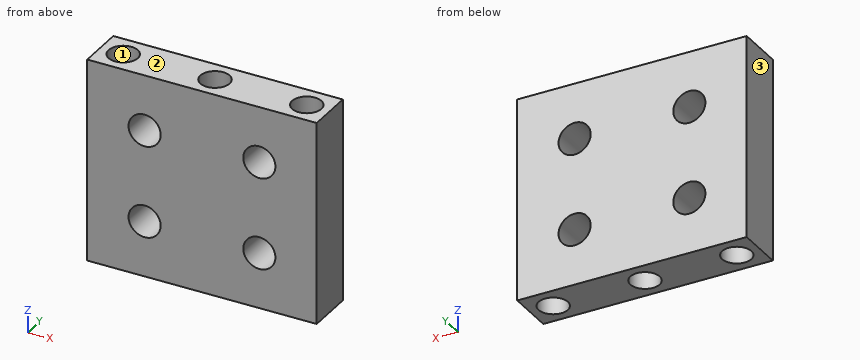
from build123d import *

# Parameters (mm, degrees)
SKETCH1_W           = 25
SKETCH1_H           = 22.12
SKETCH1_R           = 1.75
BOSS_EXTRUDE1_DEPTH = 5.13
CUT_EXTRUDE1_REACH  = 27.92
SKETCH2_R           = 1.6


with BuildPart() as part:
    # Sketch1 → Boss-Extrude1 (new body)
    with BuildSketch(Plane(origin=(0, 0, 0), x_dir=(1, 0, 0), z_dir=(0, 1, 0))):
        Rectangle(SKETCH1_W, SKETCH1_H)
        with Locations(Location((6.25, -5, 0), (0, 0, 270))):
            Circle(SKETCH1_R, mode=Mode.SUBTRACT)
        with Locations(Location((-6.25, -5, 0), (0, 0, 270))):
            Circle(SKETCH1_R, mode=Mode.SUBTRACT)
        with Locations(Location((-6.25, 5, 0), (0, 0, 270))):
            Circle(SKETCH1_R, mode=Mode.SUBTRACT)
        with Locations(Location((6.25, 5, 0), (0, 0, 270))):
            Circle(SKETCH1_R, mode=Mode.SUBTRACT)
    extrude(amount=BOSS_EXTRUDE1_DEPTH)

    # Sketch2 → Cut-Extrude1 (cut, up to next)
    with BuildSketch(Plane.XY.offset(11.06), mode=Mode.PRIVATE) as cut_extrude1_sk1:
        with Locations((0, 2.565)):
            Circle(SKETCH2_R)
    cut_extrude1_tool1 = extrude(cut_extrude1_sk1.sketch, amount=-CUT_EXTRUDE1_REACH, mode=Mode.PRIVATE) & part.part
    # Sketch2 → Cut-Extrude1 (cut, up to next)
    with BuildSketch(Plane.XY.offset(11.06), mode=Mode.PRIVATE) as cut_extrude1_sk2:
        with Locations((-10, 2.565)):
            Circle(SKETCH2_R)
    cut_extrude1_tool2 = extrude(cut_extrude1_sk2.sketch, amount=-CUT_EXTRUDE1_REACH, mode=Mode.PRIVATE) & part.part
    # Sketch2 → Cut-Extrude1 (cut, up to next)
    with BuildSketch(Plane.XY.offset(11.06), mode=Mode.PRIVATE) as cut_extrude1_sk3:
        with Locations(Location((10, 2.565, 0), (0, 0, 180))):
            Circle(SKETCH2_R)
    cut_extrude1_tool3 = extrude(cut_extrude1_sk3.sketch, amount=-CUT_EXTRUDE1_REACH, mode=Mode.PRIVATE) & part.part
    add(cut_extrude1_tool1.solids().sort_by_distance((0, 2.565, 11.06))[0], mode=Mode.SUBTRACT)
    add(cut_extrude1_tool2.solids().sort_by_distance((-10, 2.565, 11.06))[0], mode=Mode.SUBTRACT)
    add(cut_extrude1_tool3.solids().sort_by_distance((10, 2.565, 11.06))[0], mode=Mode.SUBTRACT)


solid = part.part
Verification items for the finished model (mm, model axes). Face numbers are marked on the shaded views. Coordinates: 2 decimals unless noted, no trailing zeros. Order: outer loops, then holes, each group sorted by start corner. A loop starts at its lowest first (then second) coordinate and runs counter-clockwise, first axis right, second up. Notation, with made-up numbers: M -24.5,3.5 L 15.5,3.5 A28 cw 15.5,22.5 Z; hole C -18.75,52 d6. An arc over 180 degrees is marked long. One line per item, written item: value. Start each with the question number.
Item 1: Sectioned sample at D-D (y = 1.9). Enter the section's corners in (x, z).
Item 2: Sectioned sample at A-A (x = -10). Enter the section's corners in (y, z) (3 decimals), then the cut area to 3 significant figures.
Item 3: Gauge pin test, flat ends, axial feed: pin 1 (5.5 mm diameter, centred on x = 6.25, z = 5, fed in from -Y); pin 2 (3 mm diameter, centred on x = -6.25, z = 5, fed in from -Y). Record the tip position at first contact, or that the pin passes through.
Item 4: Sectioned sample at C-C (z = 5). Enter the section's corners in (x, y) (3 decimals), then the cut area to 3 significant figures.
Item 5: Sectioned sample at B-B (x = -6.25). Enter the section's corners in (y, z), then the cut area to 3 significant figures.
Item 6: Mould release check, pull along X, two halves, no side actions. Record for the marked faces 1, 2 and 3: released by +X, released by -X, zero draft, split by the parting line, or undercut.
Item 7: Scan lines: probe 1 along X at (y, z) = (2.7, 8.25); probe 2 along X at (y, z) = (2, 10.25); probe 3 along Z at (x, y) = (4.75, 4.3). Record each from-to range of solid material in increasing order.
Conclusion:
1. outline: M -12.5,-11.06 L -11.46,-11.06 L -11.46,11.06 L -12.5,11.06 Z; M -8.54,-11.06 L -1.46,-11.06 L -1.46,11.06 L -8.54,11.06 Z; M 1.46,-11.06 L 8.54,-11.06 L 8.54,11.06 L 1.46,11.06 Z; M 11.46,-11.06 L 12.5,-11.06 L 12.5,11.06 L 11.46,11.06 Z; hole C -6.25,-5 d3.5; hole C -6.25,5 d3.5; hole C 6.25,-5 d3.5; hole C 6.25,5 d3.5
2. outline: M 0,-11.06 L 0.965,-11.06 L 0.965,11.06 L 0,11.06 Z; M 4.165,-11.06 L 5.13,-11.06 L 5.13,11.06 L 4.165,11.06 Z
2. area: 42.7 mm^2
3. pin 1: stops at y = 0
3. pin 2: passes through
4. outline: M -12.5,0 L -8,0 L -8,5.13 L -12.5,5.13 Z; M -4.5,0 L 4.5,0 L 4.5,5.13 L -4.5,5.13 Z; M 8,0 L 12.5,0 L 12.5,5.13 L 8,5.13 Z; hole C -10,2.565 d3.2; hole C 0,2.565 d3.2; hole C 10,2.565 d3.2
4. area: 68.2 mm^2
5. outline: M 0,-11.06 L 5.13,-11.06 L 5.13,-6.75 L 0,-6.75 Z; M 0,-3.25 L 5.13,-3.25 L 5.13,3.25 L 0,3.25 Z; M 0,6.75 L 5.13,6.75 L 5.13,11.06 L 0,11.06 Z
5. area: 77.6 mm^2
6. face 1: undercut
6. face 2: zero draft
6. face 3: released by -X
7. probe 1: x = -12.5 to -11.59, -8.41 to -1.59, 1.59 to 8.41, 11.59 to 12.5
7. probe 2: x = -12.5 to -11.5, -8.5 to -1.5, 1.5 to 8.5, 11.5 to 12.5
7. probe 3: z = -11.06 to -5.9, -4.1 to 4.1, 5.9 to 11.06
